```python
from build123d import *

# Parameters (mm, degrees)
SKETCH3_W                = 70
SKETCH3_H                = 20
BOSS_EXTRUDE2_DEPTH      = 5
BOSS_EXTRUDE3_DEPTH      = 15
BOSS_EXTRUDE3_DEPTH_BACK = 5
CUT_EXTRUDE1_REACH       = 7
SKETCH5_R                = 2.25
SKETCH6_R                = 3.75
CUT_EXTRUDE2_DEPTH       = 16
CUT_EXTRUDE2_DEPTH_BACK  = 1
SKETCH7_R                = 2.25
CUT_EXTRUDE3_DEPTH       = 20.85
CUT_EXTRUDE3_DEPTH_BACK  = 51.15
SKETCH11_R               = 3.75
CUT_EXTRUDE4_DEPTH       = 1
SKETCH12_R               = 3.75
CUT_EXTRUDE5_DEPTH       = 1
CHAMFER1_SIZE            = 3


with BuildPart() as part:
    # Sketch3 → Boss-Extrude2 (new body)
    with BuildSketch(Plane(origin=(0, 0, 0), x_dir=(1, 0, 0), z_dir=(0, 1, 0))):
        Rectangle(SKETCH3_W, SKETCH3_H)
    extrude(amount=BOSS_EXTRUDE2_DEPTH)

    # Sketch4 → Boss-Extrude3 (add, two sides)
    with BuildSketch(Plane(origin=(0, 5, 0), x_dir=(1, 0, 0), z_dir=(0, 1, 0))) as boss_extrude3_sk:
        Polygon((-15.15, -5), (15.15, -5), (15.15, -30), (10.15, -30), (10.15, -10), (-10.15, -10), (-10.15, -30), (-15.15, -30), align=None)
    extrude(amount=BOSS_EXTRUDE3_DEPTH)
    extrude(boss_extrude3_sk.sketch, amount=-BOSS_EXTRUDE3_DEPTH_BACK)

    # Sketch5 → Cut-Extrude1 (cut, up to next)
    with BuildSketch(Plane(origin=(0, 5, 0), x_dir=(1, 0, 0), z_dir=(0, 1, 0)), mode=Mode.PRIVATE) as cut_extrude1_sk1:
        Circle(SKETCH5_R)
    cut_extrude1_tool1 = extrude(cut_extrude1_sk1.sketch, amount=-CUT_EXTRUDE1_REACH, mode=Mode.PRIVATE) & part.part
    add(cut_extrude1_tool1.solids().sort_by_distance((0, 5, 0))[0], mode=Mode.SUBTRACT)
    # Sketch5 → Cut-Extrude1 (cut, up to next)
    with BuildSketch(Plane(origin=(0, 5, 0), x_dir=(1, 0, 0), z_dir=(0, 1, 0)), mode=Mode.PRIVATE) as cut_extrude1_sk2:
        with Locations((25, 0)):
            Circle(SKETCH5_R)
    cut_extrude1_tool2 = extrude(cut_extrude1_sk2.sketch, amount=-CUT_EXTRUDE1_REACH, mode=Mode.PRIVATE) & part.part
    add(cut_extrude1_tool2.solids().sort_by_distance((25, 5, 0))[0], mode=Mode.SUBTRACT)
    # Sketch5 → Cut-Extrude1 (cut, up to next)
    with BuildSketch(Plane(origin=(0, 5, 0), x_dir=(1, 0, 0), z_dir=(0, 1, 0)), mode=Mode.PRIVATE) as cut_extrude1_sk3:
        with Locations((-25, 0)):
            Circle(SKETCH5_R)
    cut_extrude1_tool3 = extrude(cut_extrude1_sk3.sketch, amount=-CUT_EXTRUDE1_REACH, mode=Mode.PRIVATE) & part.part
    add(cut_extrude1_tool3.solids().sort_by_distance((-25, 5, 0))[0], mode=Mode.SUBTRACT)

    # Sketch6 → Cut-Extrude2 (cut, two sides)
    with BuildSketch(Plane(origin=(0, 5, 0), x_dir=(1, 0, 0), z_dir=(0, 1, 0))) as cut_extrude2_sk:
        with Locations((-25, 0)):
            Circle(SKETCH6_R)
        Circle(SKETCH6_R)
        with Locations((25, 0)):
            Circle(SKETCH6_R)
    extrude(amount=CUT_EXTRUDE2_DEPTH, mode=Mode.SUBTRACT)
    extrude(cut_extrude2_sk.sketch, amount=-CUT_EXTRUDE2_DEPTH_BACK, mode=Mode.SUBTRACT)

    # Sketch7 → Cut-Extrude3 (cut, two sides)
    with BuildSketch(Plane.ZY.offset(15.15)) as cut_extrude3_sk:
        with Locations((20, 10)):
            Circle(SKETCH7_R)
    extrude(amount=CUT_EXTRUDE3_DEPTH, mode=Mode.SUBTRACT)
    extrude(cut_extrude3_sk.sketch, amount=-CUT_EXTRUDE3_DEPTH_BACK, mode=Mode.SUBTRACT)

    # Sketch11 → Cut-Extrude4 (cut)
    with BuildSketch(Plane.ZY.offset(15.15)):
        with Locations((20, 10)):
            Circle(SKETCH11_R)
    extrude(amount=-CUT_EXTRUDE4_DEPTH, mode=Mode.SUBTRACT)

    # Sketch12 → Cut-Extrude5 (cut)
    with BuildSketch(Plane(origin=(15.15, 0, 0), x_dir=(0, 0, -1), z_dir=(1, 0, 0))):
        with Locations((-20, 10)):
            Circle(SKETCH12_R)
    extrude(amount=-CUT_EXTRUDE5_DEPTH, mode=Mode.SUBTRACT)

    # Chamfer1
    chamfer1_edges = [part.edges().sort_by_distance(p)[0] for p in [
        (15.15, 12.5, 5),
        (-15.15, 12.5, 5),
        (-12.65, 0, 30),
        (12.65, 0, 30),
        (0, 20, 5),
        (-12.65, 20, 30),
        (12.65, 20, 30),
        (35, 2.5, 10),
        (-35, 2.5, 10),
        (-35, 2.5, -10),
        (35, 2.5, -10),
    ]]
    chamfer(chamfer1_edges, length=CHAMFER1_SIZE)


solid = part.part
```
Work out the finished part from the listing and answer in its coordinate system (mm). A direction names the side the tool comes from. Coordinates: 2 decimals unless noted, no trailing zeros. Loops run counter-clockwise (first coordinate to the right, second up) from the corner with the lowest first, then second, coordinate; pieces in that order, holes last. Notation, with made-up numbers: M -12,45.5 L 40,45.5 A16 cw 40,53.5 Z; hole C 12.25,-20 d10. An arc over 180 degrees is marked long. Use CSV: the item, a comma, the result in double quotes. Start each with the question number.
(1) Find section C-C, the plane y = 13. Give the vertices of the cut face in (x, z), then the cut area to 4 significant figures.
(2) Find section D-D, the plane x = -13. Give the vertices of the cut face in (y, z).
(3) Find section B-B, the plane z = 0. Give the vertices of the cut face in (x, y), then the cut area to 4 significant figures.
(4) For faces 1 (the face through (13.63, 12.4, 6.48)), 2 (the face through (0, 10, 10)), 3 (the face through (23, 2, 10)), 4 (the face through (-24, 2, 10)), 5 (the face through (2, 4, 2)), determine the directions among +Z, -Z, +X, -X, +Y, -Y from which every point of the face is accessible in a straight line to the end or side of a thin tool.
(5) Consider line 1 (X direction, y = 0.9, z = 0); line 2 (Z direction, x = -25, y = 1.15); line 3 (X direction, y = 7.5, z = 21). Determine where each line is inside the solid, lowest interval first.
(6) Find section A-A, the plane x = 0. Give the vertices of the cut face in (y, z), then the cut area to 3 significant figures.
(7) Given pin 1 Ø1.5 at (y, z) = (6, 17.5) entering from -X; pin 2 Ø6 at (x, z) = (1.5, 1) entering from +Y; pin 3 Ø2.5 at (x, z) = (-25, 0) entering from -Y; pin 4 Ø10 at (x, y) = (25.5, 5.5) entering from +Z, each flat-ended and moving along its own axis, determine where each tip first touches the part or whether it passes through.
(8) For a pull along Y with two mould halves and no side action, classify faces 6 (the face through (-12.178, 10.676, 22.146)), 7 (the face through (-13, 2, 29)), 8 (the face through (-14.657, 13.718, 19.512)), 9 (the face through (13, 10, 30)) as +Y half, -Y half, draft (parallel to the pull), parting line (faces both ways), or undercut.
Recorded:
1,outline,"M -15.15,8 L -12.15,5 L 12.15,5 L 15.15,8 L 15.15,17.75 L 14.15,17.75 L 14.15,22.25 L 15.15,22.25 L 15.15,30 L 10.15,30 L 10.15,10 L -10.15,10 L -10.15,30 L -15.15,30 L -15.15,22.25 L -14.15,22.25 L -14.15,17.75 L -15.15,17.75 Z"
1,area,"333.5 mm^2"
2,outline,"M 0,-10 L 5,-10 L 5,5.85 L 17.85,5.85 L 20,8 L 20,27 L 17,30 L 3,30 L 0,27 Z; hole C 10,20 d4.5"
3,outline,"M -35,0 L -27.25,0 L -27.25,4 L -28.75,4 L -28.75,5 L -35,5 Z; M -22.75,0 L -2.25,0 L -2.25,4 L -3.75,4 L -3.75,5 L -21.25,5 L -21.25,4 L -22.75,4 Z; M 2.25,0 L 22.75,0 L 22.75,4 L 21.25,4 L 21.25,5 L 3.75,5 L 3.75,4 L 2.25,4 Z; M 27.25,0 L 35,0 L 35,5 L 28.75,5 L 28.75,4 L 27.25,4 Z"
3,area,"273.5 mm^2"
4,face 1,"-Z, +X, +Y"
4,face 2,"+Z, +Y, -Y"
4,face 3,"+Z, +X, +Y, -Y"
4,face 4,"+Z, -X, +Y, -Y"
4,face 5,"+Y"
5,line 1,"x = -35 to -27.25, -22.75 to -2.25, 2.25 to 22.75, 27.25 to 35"
5,line 2,"z = -10 to -2.25, 2.25 to 10"
5,line 3,"x = -14.15 to -10.15, 10.15 to 14.15"
6,outline,"M 0,-10 L 5,-10 L 5,-3.75 L 4,-3.75 L 4,-2.25 L 0,-2.25 Z; M 0,2.25 L 4,2.25 L 4,3.75 L 5,3.75 L 5,5 L 17,5 L 20,8 L 20,10 L 0,10 Z"
6,area,"145 mm^2"
7,pin 1,"stops at x = -15.15"
7,pin 2,"stops at y = 5"
7,pin 3,"passes through"
7,pin 4,"stops at z = 10"
8,face 6,"undercut"
8,face 7,"-Y half"
8,face 8,"undercut"
8,face 9,"draft"
